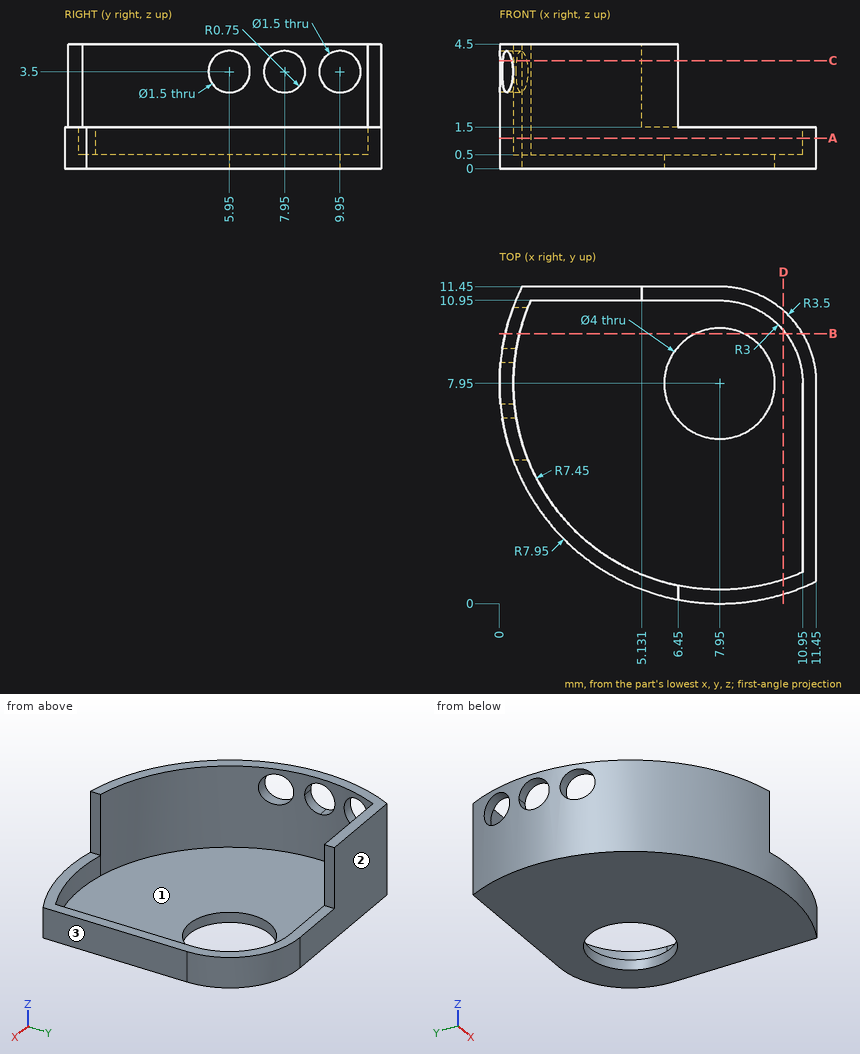
Study the drawing (mm; zero at the part's minimum x, y, z) and answer. Give positions to 0.01 mm unless a question says otherwise; leave off trailing zeros. Loops run counter-clockwise (first coordinate to the right, second up) from the corner with the lowest first, then second, coordinate; pieces in that order, holes last. Notation, with made-up numbers: (-2.75, 28) - (15.25, 28) arc R36 ccw to (15.25, 64) - close; hole circle Ø8 at (-18, 9.25). An arc over 180 degrees is marked (long way). Answer in a Markdown table with one row per item. Add a question column.
Q1. The part is cut by section D-D (x = 10.25). Determine the outline of the cut face in (y, z).
Q2. Each of these flat-tipped pins is pushed along its axis until it touches: P1, Ø1.5, axis at y = 4, z = 2.5, coming from the -X side; P2, Ø1.7, axis at y = 5.95, z = 3.5, coming from the -X side; P3, Ø1.9, axis at x = 9.5, y = 5, coming from the +Z side. Where does it stop, or does it pass through?
Q3. Consider line 1 along Z through (x, y) = (0.7, 5.95); line 2 along Z through (x, y) = (2.25, 10.25); line 3 along Y through (x, z) = (4.5, 2.2). Determine where each line is inside the solid, lowest interval first.
Q4. The part is cut by section A-A (z = 1.1). Determine the outline of the cut face in (x, y).
Q5. The part is cut by section C-C (z = 3.9). State how many separate pieces and enclosed holes the cut face has.
Q6. The part is cut by section B-B (y = 9.75). Determine the outline of the cut face in (x, z).
Q7. Determine the mould class of the marked faces 1, 2 and 3 for opening direction X: released by +X, released by -X, zero draft, split by the parting line, or undercut.
Solution:
| question | item | result |
|---|---|---|
| 1 | outline | (0.34, 0) - (10.59, 0) - (10.59, 1.5) - (9.88, 1.5) - (9.88, 0.5) - (0.86, 0.5) - (0.86, 1.5) - (0.34, 1.5) - close |
| 2 | P1 | stops at x = 0.67 |
| 2 | P2 | stops at x = 0.08 |
| 2 | P3 | stops at z = 0.5 |
| 3 | line 1 | z = 0 to 2.75, 4.25 to 4.5 |
| 3 | line 2 | z = 0 to 0.5 |
| 3 | line 3 | y = 0.79 to 1.35, 10.95 to 11.45 |
| 4 | outline | (0.81, 11.45) arc R7.95 ccw to (11.45, 0.81) - (11.45, 7.95) arc R3.5 ccw to (7.95, 11.45) - close; hole (1.13, 10.95) arc R7.45 ccw to (10.95, 1.13) - (10.95, 7.95) arc R3 ccw to (7.95, 10.95) - close |
| 5 | separate pieces | 4 |
| 5 | enclosed holes | 0 |
| 6 | outline | (0.21, 0) - (7.08, 0) - (7.08, 0.5) - (0.72, 0.5) - (0.72, 2.78) - (0.21, 2.78) - close; (0.21, 4.22) - (0.72, 4.22) - (0.72, 4.5) - (0.21, 4.5) - close; (8.82, 0) - (10.95, 0) - (10.95, 1.5) - (10.35, 1.5) - (10.35, 0.5) - (8.82, 0.5) - close |
| 7 | face 1 | undercut |
| 7 | face 2 | zero draft |
| 7 | face 3 | released by +X |
